```python
from build123d import *

# Parameters (mm, degrees)
F0_W     = 69.85
F0_H     = 69.85
F1_DEPTH = 16.891
F2_R     = 2.54
F3_DEPTH = 16.892
F4_R     = 3.175
F5_DEPTH = 16.892


with BuildPart() as f1:
    # F0 (on Top) → F1 (new body)
    with BuildSketch(Plane.XY):
        Rectangle(F0_W, F0_H)
    extrude(amount=F1_DEPTH)

    # F2 (on face) → F3 (cut, through all)
    with BuildSketch(Plane.XY.offset(16.891)):
        with Locations((-22.9997, 6.5024)):
            Circle(F2_R)
        with Locations((22.9997, 6.5024)):
            Circle(F2_R)
        with Locations((22.9997, -6.5024)):
            Circle(F2_R)
        with Locations((-22.9997, -6.5024)):
            Circle(F2_R)
    extrude(amount=-F3_DEPTH, mode=Mode.SUBTRACT)

    # F4 (on face) → F5 (cut, through all)
    with BuildSketch(Plane.XY.offset(16.891)):
        with Locations((-25.4, 25.4)):
            Circle(F4_R)
        with Locations((25.4, 25.4)):
            Circle(F4_R)
        with Locations((-25.4, -25.4)):
            Circle(F4_R)
        with Locations((25.4, -25.4)):
            Circle(F4_R)
    extrude(amount=-F5_DEPTH, mode=Mode.SUBTRACT)


solid = f1.part
```
CAD build for the part. Positions are in the model's coordinates, mm. Coordinates: 2 decimals unless noted, no trailing zeros. Order: outer loops, then holes, each group sorted by start corner. A loop starts at its lowest first (then second) coordinate and runs counter-clockwise, first axis right, second up.
(1) Saw through at A-A, the plane y = -25.4. Write the cut outline in (x, z) (3 decimals).
Solution:
outline: (-34.925, 0) - (-28.575, 0) - (-28.575, 16.891) - (-34.925, 16.891) - close; (-22.225, 0) - (22.225, 0) - (22.225, 16.891) - (-22.225, 16.891) - close; (28.575, 0) - (34.925, 0) - (34.925, 16.891) - (28.575, 16.891) - close
(2) Saw through at B-B, the plane z = 8.5. Count the separate pieces of the cut face and the enclosed holes in it, and give its area (3 significant figures).
Solution:
separate pieces: 1
enclosed holes: 8
area: 4,670 mm2
(3) Pin check, flat tips, straight feed: pin 1 Ø8.5 at (x, y) = (25.4, -25.4) entering from -Z; pin 2 Ø3 at (x, y) = (23, 6.5) entering from +Z. Stop position of each tip, or through.
Solution:
pin 1: stops at z = 0
pin 2: passes through
(4) Mould opens along X. For faces 1 (the face through (-34.925, 0, 8)), 2 (the face through (0, 0, 0)), 3 (the face through (34.925, 0, 8)), 4 (the face through (-25.537, 6.614, 8.564)) say: released by +X, released by -X, zero draft, split by the parting line, or undercut.
Solution:
face 1: released by -X
face 2: zero draft
face 3: released by +X
face 4: undercut
(5) Drill centre lines: L1, parallel to Y at x = -24, z = 14.75 (3 decimals); L2, parallel to X at y = 7, z = 2.5 (3 decimals); L3, parallel to X at y = 28, z = 1 (3 decimals). Where is each one in solid material? Low to high.
Solution:
L1: y = -34.925 to -28.25, -22.55 to -8.837, -4.168 to 4.168, 8.837 to 22.55, 28.25 to 34.925
L2: x = -34.925 to -25.49, -20.509 to 20.509, 25.49 to 34.925
L3: x = -34.925 to -27.222, -23.578 to 23.578, 27.222 to 34.925
